Can you work these out from the model? Positions are in its coordinate system, mm. A direction names the side the tool comes from. Round coordinates to 2 decimals unless told otherwise and drop trailing zeros. Order: outer loops, then holes, each group sorted by start corner. A loop starts at its lowest first (then second) coordinate and runs counter-clockwise, first axis right, second up. Notation, with made-up numbers: M 35,38 L 87,38 A22 cw 87,72 Z; hole C 57,-21.75 d8. An arc over 180 degrees is marked long. Answer as CSV lines item,"result". Start each with the question number.
from build123d import *

# Parameters (mm, degrees)
SKETCH2_R           = 8.5
BOSS_EXTRUDE1_DEPTH = 5


with BuildPart() as part:
    # Sketch2 → Boss-Extrude1 (new body)
    with BuildSketch(Plane(origin=(0, 0, 0), x_dir=(0, 0, -1), z_dir=(1, 0, 0))):
        Polygon((-50, -12.5), (-40, -12.5), (-40, -17.5), (-25, -17.5), (-25, -12.5), (25, -12.5), (25, -17.5), (40, -17.5), (40, -12.5), (50, -12.5), (50, 12.5), (40, 12.5), (40, 17.5), (25, 17.5), (25, 12.5), (-25, 12.5), (-25, 17.5), (-40, 17.5), (-40, 12.5), (-50, 12.5), align=None)
        with Locations((-13, 0)):
            Circle(SKETCH2_R, mode=Mode.SUBTRACT)
        with Locations(Location((13, 0, 0), (0, 0, 180))):
            Circle(SKETCH2_R, mode=Mode.SUBTRACT)
    extrude(amount=BOSS_EXTRUDE1_DEPTH)


solid = part.part
(1) I want a section at A-A on y = 14. Write out the boundary of the cut face in (x, z), and give its area (3 significant figures).
(2) I want a section at B-B on z = 13. Write out the boundary of the cut face in (x, y), and give its area (3 significant figures).
(3) I'm going to push flat-ended pins straight in: P1, Ø2.5, axis at x = 1.5, y = -14, coming from the -Z side; P2, Ø2.5, axis at x = 2, y = -14.5, coming from the +Z side; P3, Ø1.5, axis at x = 3, z = -4, coming from the -Y side. Where does each tip first touch, or does it pass through?
(4) For faces 1 (the flat face through (2, -15, 25)), 2 (the flat face through (2, 12.5, 45)), 3 (the flat face through (2, 15, 25)), which set-ups out of +Z, -Z, +X, -X, +Y, -Y let a thin tool reach every point of the face, with its end or its side?
(5) I want a section at C-C on x = 2.95. Write out the boundary of the cut face in (y, z), and give its area (3 significant figures).
(6) If we mould it in two halves opening along Y, with no side actions, what happens to faces 4 (the flat face through (5, 0, 1)), 5 (the flat face through (2, -12.5, 45)), 6 (the cylindrical face through (2.465, 5.745, 19.265))? For each: +Y half, -Y half, draft (parallel to the pull), parting line (faces both ways), or undercut.
(7) If I drill on line 1 along Y through (x, z) = (3.3, 13); line 2 along Z through (x, y) = (2.7, -6); line 3 along Z through (x, y) = (0.3, 14), over which ranges is the centre line in solid material (lowest first)?
(8) I want a section at D-D on y = 0. Write out the boundary of the cut face in (x, z).
From the geometry:
1,outline,"M 0,-40 L 5,-40 L 5,-25 L 0,-25 Z; M 0,25 L 5,25 L 5,40 L 0,40 Z"
1,area,"150 mm²"
2,outline,"M 0,-12.5 L 5,-12.5 L 5,-8.5 L 0,-8.5 Z; M 0,8.5 L 5,8.5 L 5,12.5 L 0,12.5 Z"
2,area,"40.0 mm²"
3,P1,"z = -40"
3,P2,"z = 40"
3,P3,"y = -12.5"
4,face 1,"+X, -X, -Y"
4,face 2,"+Z, +X, -X, +Y"
4,face 3,"+X, -X, +Y"
5,outline,"M -17.5,-40 L -12.5,-40 L -12.5,-50 L 12.5,-50 L 12.5,-40 L 17.5,-40 L 17.5,-25 L 12.5,-25 L 12.5,25 L 17.5,25 L 17.5,40 L 12.5,40 L 12.5,50 L -12.5,50 L -12.5,40 L -17.5,40 L -17.5,25 L -12.5,25 L -12.5,-25 L -17.5,-25 Z; hole C 0,-13 d17; hole C 0,13 d17"
5,area,"2,350 mm²"
6,face 4,"draft"
6,face 5,"-Y half"
6,face 6,"undercut"
7,line 1,"-12.5 to -8.5, 8.5 to 12.5"
7,line 2,"-50 to -19.02, -6.98 to 6.98, 19.02 to 50"
7,line 3,"-40 to -25, 25 to 40"
8,outline,"M 0,-50 L 5,-50 L 5,-21.5 L 0,-21.5 Z; M 0,-4.5 L 5,-4.5 L 5,4.5 L 0,4.5 Z; M 0,21.5 L 5,21.5 L 5,50 L 0,50 Z"
